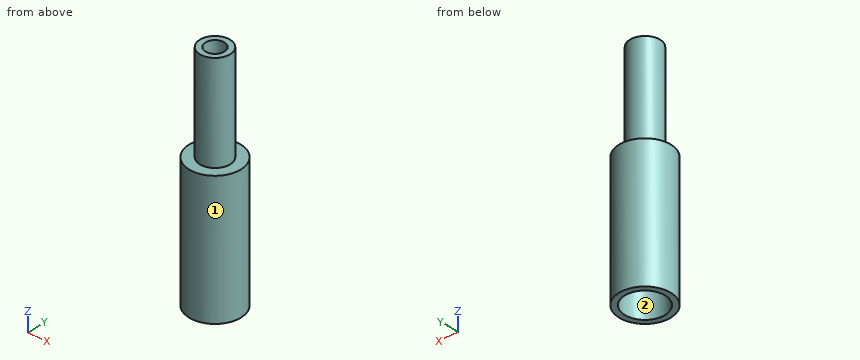
```python
from build123d import *

# Parameters (mm, degrees)
F0_R     = 13.75
F1_DEPTH = 70
F2_R     = 8.05
F3_DEPTH = 52
F4_R     = 10.75
F5_DEPTH = 52
F6_R     = 5.05
F7_DEPTH = 70


with BuildPart() as f1:
    # F0 (on Top) → F1 (new body)
    with BuildSketch(Plane.XY):
        Circle(F0_R)
    extrude(amount=F1_DEPTH)

    # F2 (on face) → F3 (join)
    with BuildSketch(Plane.XY.offset(70)):
        Circle(F2_R)
    extrude(amount=F3_DEPTH)

    # F4 (on face) → F5 (cut)
    with BuildSketch(Plane(origin=(0, 0, 0), x_dir=(1, 0, 0), z_dir=(0, 0, -1))):
        Circle(F4_R)
    extrude(amount=-F5_DEPTH, mode=Mode.SUBTRACT)

    # F6 (on face) → F7 (cut, through all)
    with BuildSketch(Plane.XY.offset(122)):
        Circle(F6_R)
    extrude(amount=-F7_DEPTH, mode=Mode.SUBTRACT)


solid = f1.part
```
The listing builds one solid part. Answer for the finished solid, in the listing's coordinates (mm). Face numbers are marked on the shaded views. Give positions to 0.01 mm unless a question says otherwise; leave off trailing zeros. Order: outer loops, then holes, each group sorted by start corner. A loop starts at its lowest first (then second) coordinate and runs counter-clockwise, first axis right, second up.
1) Find section A-A on x = 0. Write down the section's boundary in (y, z), then the cut area to 3 significant figures.
Reported:
outline: (-13.75, 0) - (-10.75, 0) - (-10.75, 52) - (-5.05, 52) - (-5.05, 122) - (-8.05, 122) - (-8.05, 70) - (-13.75, 70) - close; (5.05, 52) - (10.75, 52) - (10.75, 0) - (13.75, 0) - (13.75, 70) - (8.05, 70) - (8.05, 122) - (5.05, 122) - close
area: 937 mm2
2) Find section C-C on z = 68.5. Write down the section's boundary in (x, y), then the cut area to 3 significant figures.
Reported:
outline: circle Ø27.5 at (0, 0); hole circle Ø10.1 at (0, 0)
area: 514 mm2
3) Find section D-D on y = -6.5. Write down the section's boundary in (x, z).
Reported:
outline: (-12.12, 0) - (-8.56, 0) - (-8.56, 52) - (8.56, 52) - (8.56, 0) - (12.12, 0) - (12.12, 70) - (4.75, 70) - (4.75, 122) - (-4.75, 122) - (-4.75, 70) - (-12.12, 70) - close
4) Consider line 1 along Y through (x, z) = (0.5, 76); line 2 along Y through (x, z) = (0, 37.5); line 3 along Z through (x, y) = (-7.5, -9). Determine where each line is inside the solid, lowest interval first.
Reported:
line 1: y = -8.03 to -5.03, 5.03 to 8.03
line 2: y = -13.75 to -10.75, 10.75 to 13.75
line 3: z = 0 to 70
5) Determine the mould class of the marked faces 1 and 2 for opening direction Y: pulls with the +Y half, pulls with the -Y half, needs draft (parallel to the pull), parting line crosses it, or undercut.
Reported:
face 1: parting line crosses it
face 2: undercut
6) Given P1, Ø8, axis at x = -10, z = 104.5, coming from the +Y side; P2, Ø2, axis at y = -11, z = 68, coming from the +X side; P3, Ø4, axis at y = -6.5, z = 30.5, coming from the -X side, each flat-ended and moving along its own axis, determine where each tip first touches the part or whether it passes through.
Reported:
P1: stops at y = 5.37
P2: stops at x = 9.44
P3: stops at x = -12.99
